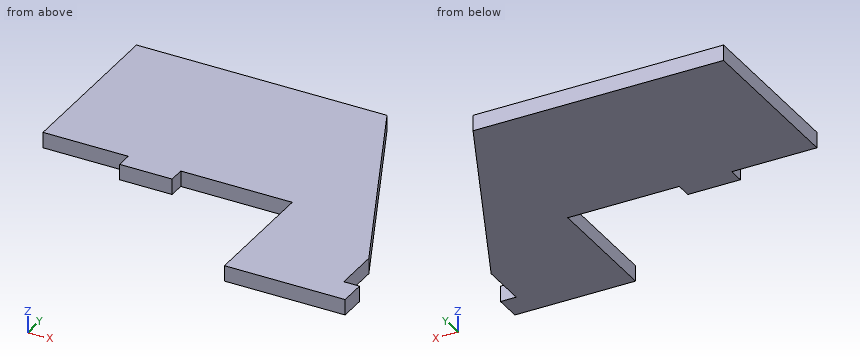
from build123d import *

# Parameters (mm, degrees)
ESQUISSE1_W             = 135
ESQUISSE1_H             = 112.17
BOSS_EXTRU_1_DEPTH      = 6
ENL_V_MAT_EXTRU_1_DEPTH = 6
ESQUISSE3_W             = 6
ESQUISSE3_H             = 10
ESQUISSE3_W_2           = 20
ESQUISSE3_H_2           = 6
BOSS_EXTRU_2_DEPTH      = 6


with BuildPart() as part:
    # Esquisse1 → Boss.-Extru.1 (new body)
    with BuildSketch(Plane.XY):
        Rectangle(ESQUISSE1_W, ESQUISSE1_H)
    extrude(amount=BOSS_EXTRU_1_DEPTH)

    # Esquisse2 → Enlèv. mat.-Extru.1 (cut)
    with BuildSketch(Plane.XY.offset(6)):
        Polygon((27.5, -56.085), (-67.5, -56.085), (-67.5, -8.915), (-38.5, -8.915), (27.5, -8.915), align=None)
        Polygon((67.5, -28.665), (27.980425971, 56.085), (67.5, 56.085), align=None)
    extrude(amount=-ENL_V_MAT_EXTRU_1_DEPTH, mode=Mode.SUBTRACT)

    # Esquisse3 → Boss.-Extru.2 (add)
    with BuildSketch(Plane.XY.offset(6)):
        with Locations((70.5, -51.085)):
            Rectangle(ESQUISSE3_W, ESQUISSE3_H)
        with Locations((-25, -11.915)):
            Rectangle(ESQUISSE3_W_2, ESQUISSE3_H_2)
    extrude(amount=-BOSS_EXTRU_2_DEPTH)


solid = part.part
Geometry check sheet. Reference: the model listing, model coordinates, mm. Give positions to 0.01 mm unless a question says otherwise; leave off trailing zeros. Order: outer loops, then holes, each group sorted by start corner. A loop starts at its lowest first (then second) coordinate and runs counter-clockwise, first axis right, second up.
1. Sectioned sample at A-A (z = 2.55). Record the boundary of the cut face in (x, y) (3 decimals).
Completed:
outline: (-67.5, -8.915) - (-35, -8.915) - (-35, -14.915) - (-15, -14.915) - (-15, -8.915) - (27.5, -8.915) - (27.5, -56.085) - (73.5, -56.085) - (73.5, -46.085) - (67.5, -46.085) - (67.5, -28.665) - (27.98, 56.085) - (-67.5, 56.085) - close
2. Depth check by flat-ended pin: pin 1 (1.8 mm diameter, centred on x = 6.5, z = 1.5, fed in from -Y) (3 decimals); pin 2 (2 mm diameter, centred on x = 43, y = 26.5, fed in from +Z); pin 3 (1.8 mm diameter, centred on y = -33.5, z = 2, fed in from +X); pin 4 (2 mm diameter, centred on y = -31.5, z = 2, fed in from -X). Enter the tip coordinate at first touch or a pass-through.
Completed:
pin 1: stops at y = -8.915
pin 2: passes through
pin 3: stops at x = 67.5
pin 4: stops at x = 27.5
3. Sectioned sample at B-B (x = -48). Record the boundary of the cut face in (y, z) (3 decimals).
Completed:
outline: (-8.915, 0) - (56.085, 0) - (56.085, 6) - (-8.915, 6) - close
4. Sectioned sample at C-C (y = -49). Record the boundary of the cut face in (x, z), then the cut area to 3 significant figures.
Completed:
outline: (27.5, 0) - (73.5, 0) - (73.5, 6) - (27.5, 6) - close
area: 276 mm2
5. Scan lines: line 1 (Y direction, x = -57, z = 2.05) (3 decimals); line 2 (Y direction, x = -32, z = 0.75) (3 decimals); line 3 (X direction, y = -46.5, z = 1.1). Record each from-to range of solid material in increasing order.
Completed:
line 1: y = -8.915 to 56.085
line 2: y = -14.915 to 56.085
line 3: x = 27.5 to 73.5
